Geometry: final body of the model. Coordinates: model frame, mm. Face numbers are marked on the shaded views. A direction names the side the tool comes from. Round coordinates to 2 decimals unless told otherwise and drop trailing zeros. Write each loop counter-clockwise with the first axis right and the second up, starting at its lowest first coordinate (ties: lowest second). Pieces come first, ordered by that corner, then holes. Notation, with made-up numbers: (68, 54) - (125, 54) arc R27 cw to (125, 81) - close; hole circle Ø5 at (-16.5, 48). An arc over 180 degrees is marked (long way). Write each question's results on one line, items separated by ' | '.
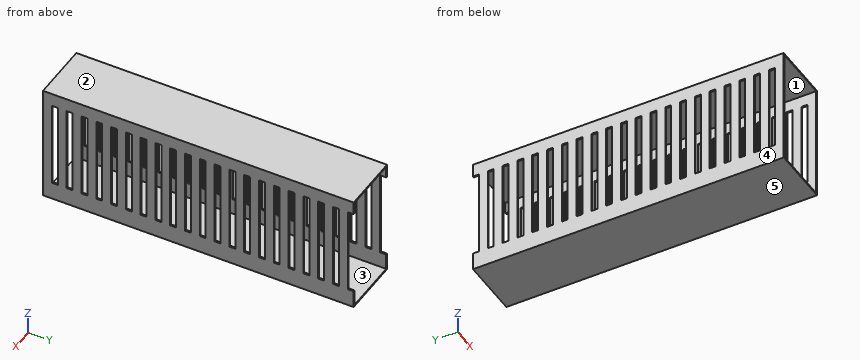
from build123d import *

# Parameters (mm, degrees)
F1_W     = 40
F1_H     = 80
F2_DEPTH = 210
F3_T     = -1
F4_W     = 4
F4_H     = 59
F5_DEPTH = 40.001


with BuildPart() as f2:
    # F1 (on Front) → F2 (new body)
    with BuildSketch(Plane.XZ):
        Rectangle(F1_W, F1_H)
    extrude(amount=F2_DEPTH)

    # F3
    f3_openings = [f2.faces().sort_by_distance(p)[0] for p in [
        (0, -210, 0),
        (0, 0, 0),
    ]]
    offset(amount=F3_T, openings=f3_openings)

    # F4 (on face) → F5 (cut, through all)
    with BuildSketch(Plane.YZ.offset(20)):
        with Locations((-202, 1.5)):
            Rectangle(F4_W, F4_H)
        with Locations((-192, 1.5)):
            Rectangle(F4_W, F4_H)
        with Locations((-182, 1.5)):
            Rectangle(F4_W, F4_H)
        with Locations((-172, 1.5)):
            Rectangle(F4_W, F4_H)
        with Locations((-162, 1.5)):
            Rectangle(F4_W, F4_H)
        with Locations((-152, 1.5)):
            Rectangle(F4_W, F4_H)
        with Locations((-142, 1.5)):
            Rectangle(F4_W, F4_H)
        with Locations((-132, 1.5)):
            Rectangle(F4_W, F4_H)
        with Locations((-122, 1.5)):
            Rectangle(F4_W, F4_H)
        with Locations((-112, 1.5)):
            Rectangle(F4_W, F4_H)
        with Locations((-102, 1.5)):
            Rectangle(F4_W, F4_H)
        with Locations((-92, 1.5)):
            Rectangle(F4_W, F4_H)
        with Locations((-82, 1.5)):
            Rectangle(F4_W, F4_H)
        with Locations((-72, 1.5)):
            Rectangle(F4_W, F4_H)
        with Locations((-62, 1.5)):
            Rectangle(F4_W, F4_H)
        with Locations((-52, 1.5)):
            Rectangle(F4_W, F4_H)
        with Locations((-42, 1.5)):
            Rectangle(F4_W, F4_H)
        with Locations((-32, 1.5)):
            Rectangle(F4_W, F4_H)
        with Locations((-22, 1.5)):
            Rectangle(F4_W, F4_H)
        with Locations((-12, 1.5)):
            Rectangle(F4_W, F4_H)
        with Locations((-2, 1.5)):
            Rectangle(F4_W, F4_H)
        with Locations((8, 1.5)):
            Rectangle(F4_W, F4_H)
        with Locations((18, 1.5)):
            Rectangle(F4_W, F4_H)
        with Locations((28, 1.5)):
            Rectangle(F4_W, F4_H)
        with Locations((38, 1.5)):
            Rectangle(F4_W, F4_H)
        with Locations((48, 1.5)):
            Rectangle(F4_W, F4_H)
        with Locations((58, 1.5)):
            Rectangle(F4_W, F4_H)
        with Locations((68, 1.5)):
            Rectangle(F4_W, F4_H)
        with Locations((78, 1.5)):
            Rectangle(F4_W, F4_H)
        with Locations((88, 1.5)):
            Rectangle(F4_W, F4_H)
        with Locations((98, 1.5)):
            Rectangle(F4_W, F4_H)
        with Locations((108, 1.5)):
            Rectangle(F4_W, F4_H)
        with Locations((118, 1.5)):
            Rectangle(F4_W, F4_H)
        with Locations((128, 1.5)):
            Rectangle(F4_W, F4_H)
        with Locations((138, 1.5)):
            Rectangle(F4_W, F4_H)
        with Locations((148, 1.5)):
            Rectangle(F4_W, F4_H)
        with Locations((158, 1.5)):
            Rectangle(F4_W, F4_H)
        with Locations((168, 1.5)):
            Rectangle(F4_W, F4_H)
        with Locations((178, 1.5)):
            Rectangle(F4_W, F4_H)
        with Locations((198, 1.5)):
            Rectangle(F4_W, F4_H)
        with Locations((208, 1.5)):
            Rectangle(F4_W, F4_H)
        with Locations((218, 1.5)):
            Rectangle(F4_W, F4_H)
        with Locations((228, 1.5)):
            Rectangle(F4_W, F4_H)
        with Locations((238, 1.5)):
            Rectangle(F4_W, F4_H)
        with Locations((188, 1.5)):
            Rectangle(F4_W, F4_H)
    extrude(amount=-F5_DEPTH, mode=Mode.SUBTRACT)


solid = f2.part
Q1. Mould query, pull axis Z, two halves, no side actions, for the marked faces 3, 4 and 5. Classes: pulls with the +Z half, pulls with the -Z half, needs draft (parallel to the pull), parting line crosses it, or undercut.
Answer block:
face 3: undercut | face 4: needs draft | face 5: pulls with the -Z half
Q2. Pin query (flat end, axial travel): pin 1 (1.1 mm diameter, centred on x = 19.5, z = 15, fed in from +Y). Return the tip coordinate at first contact, or that it passes through.
Answer block:
pin 1: y = -4
Q3. Section query C-C, the plane y = -136. Return loops of the section in (x, z), plus the area to 3 significant figures.
Answer block:
outline: (-20, -40) - (20, -40) - (20, 40) - (-20, 40) - close; hole (-19, -39) - (19, -39) - (19, 39) - (-19, 39) - close | area: 236 mm2
Q4. Ray query, line 1 along X through (y, z) = (-104.5, 33); line 2 along Z through (x, y) = (-15, -194). Return the intervals inside material, ascending.
Answer block:
line 1: -20 to -19, 19 to 20 | line 2: -40 to -39, 39 to 40
Q5. Section query A-A, the plane x = -5. Return loops of the section in (y, z).
Answer block:
outline: (-210, -40) - (0, -40) - (0, -39) - (-210, -39) - close; (-210, 39) - (0, 39) - (0, 40) - (-210, 40) - close
Q6. Section query B-B, the plane z = -32.5. Return loops of the section in (x, y).
Answer block:
outline: (-20, -210) - (-19, -210) - (-19, 0) - (-20, 0) - close; (19, -210) - (20, -210) - (20, 0) - (19, 0) - close
Q7. Access query for the marked faces 1 and 2. Directions: +Z, -Z, +X, -X, +Y, -Y. A direction counts if a zero-diameter tool reaches every point of the face in a straight line with its end or side. Return the directions, or none.
Answer block:
face 1: +Y, -Y | face 2: +Z, +X, -X, +Y, -Y
